Check sheet for the drawn part. Datum: minimum x, y, z corner. Units: mm. A direction names the side the tool comes from. Round coordinates to 2 decimals unless told otherwise and drop trailing zeros. Write each loop counter-clockwise with the first axis right and the second up, starting at its lowest first coordinate (ties: lowest second). Pieces come first, ordered by that corner, then holes.
Item 1: Tool access check on the marked faces 5, 6 and 7. Record the directions out of +Z, -Z, +X, -X, +Y, -Y that give a thin tool (end or side, any length) a straight path to the whole face; none if there is none.
Item 2: Release check for a two-part mould opening along Z. For the marked faces 1, 2, 3 and 4 record: +Z half, -Z half, draft (parallel to the pull), parting line (faces both ways), or undercut.
Item 3: Go/stop test with flat-tipped pins: pin 1 Ø5 at (y, z) = (25, 65) entering from +X; pin 2 Ø10 at (y, z) = (25, 39) entering from +X; pin 3 Ø19 at (x, z) = (45, 79.5) entering from -Y; pin 4 Ø10 at (x, z) = (41.275, 76.2) entering from +Y. Record where each tip stops, or that it passes through.
Item 4: Cross-section at A-A on y = 38.1. Enter the section's corners in (x, z) (3 decimals).
Item 5: Material ranges on line 1 (Y direction, x = 139.7, z = 6.75); line 2 (X direction, y = 38, z = 25); line 3 (X direction, y = 38.1, z = 12.25), recorded low to high.
Item 6: Cross-section at C-C on y = 5. Enter the section's corners in (x, z) (3 decimals).
Item 7: Cross-section at D-D on z = 76.2. Enter the section's corners in (x, y) (3 decimals), plus the area to 3 significant figures.
Item 8: Cross-section at B-B on x = 139.7. Enter the section's corners in (y, z) (3 decimals), plus the area to 3 significant figures.
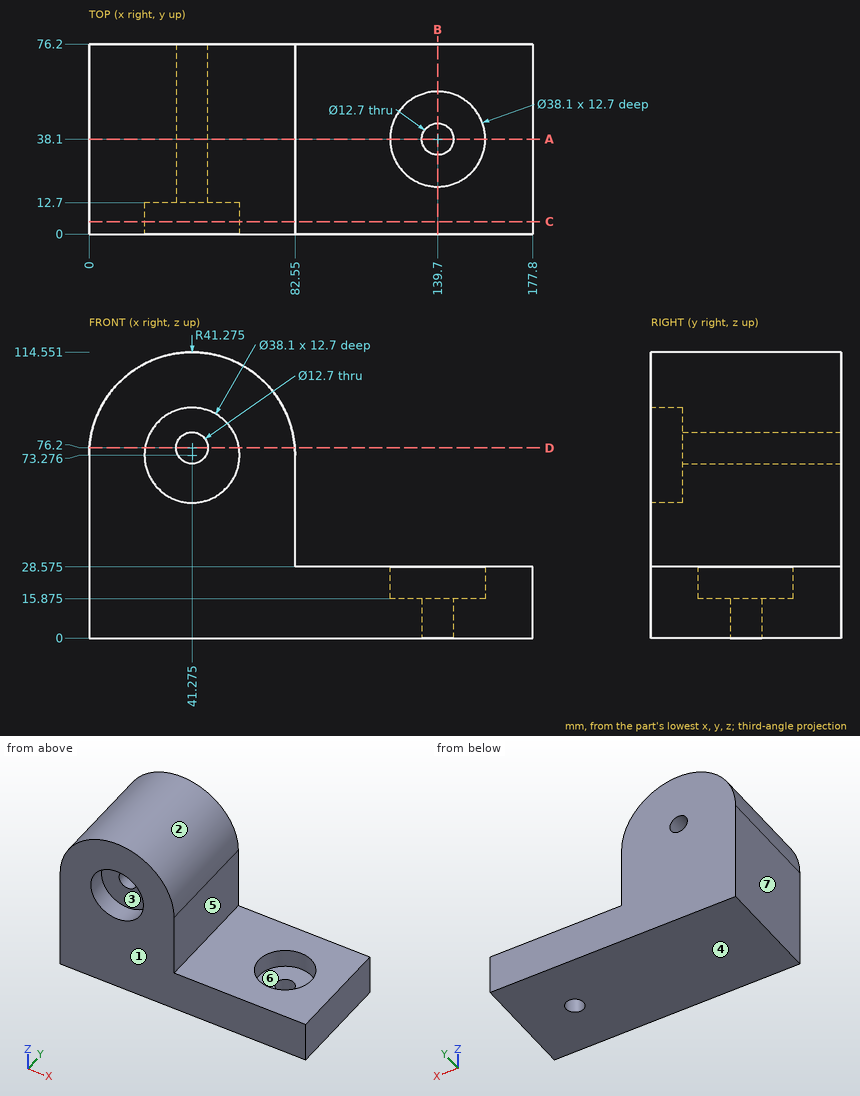
Response values:
1. face 5: +Z, +X, +Y, -Y
1. face 6: +Z
1. face 7: +Z, -Z, -X, +Y, -Y
2. face 1: draft
2. face 2: +Z half
2. face 3: undercut
2. face 4: -Z half
3. pin 1: stops at x = 82.55
3. pin 2: stops at x = 82.55
3. pin 3: stops at y = 12.7
3. pin 4: passes through
4. outline: (0, 0) - (133.35, 0) - (133.35, 15.875) - (120.65, 15.875) - (120.65, 28.575) - (82.55, 28.575) - (82.55, 73.276) arc R41.275 ccw to (0, 73.276) - close; (146.05, 0) - (177.8, 0) - (177.8, 28.575) - (158.75, 28.575) - (158.75, 15.875) - (146.05, 15.875) - close; hole circle Ø12.7 at (41.275, 76.2)
5. line 1: y = 0 to 31.75, 44.45 to 76.2
5. line 2: x = 0 to 120.65, 158.75 to 177.8
5. line 3: x = 0 to 133.35, 146.05 to 177.8
6. outline: (0, 0) - (177.8, 0) - (177.8, 28.575) - (82.55, 28.575) - (82.55, 73.276) arc R41.275 ccw to (0, 73.276) - close; hole circle Ø38.1 at (41.275, 73.276)
7. outline: (0.104, 0) - (22.451, 0) - (22.451, 12.7) - (34.925, 12.7) - (34.925, 76.2) - (0.104, 76.2) - close; (47.625, 12.7) - (60.099, 12.7) - (60.099, 0) - (82.446, 0) - (82.446, 76.2) - (47.625, 76.2) - close
7. area: 4,990 mm2
8. outline: (0, 0) - (31.75, 0) - (31.75, 15.875) - (19.05, 15.875) - (19.05, 28.575) - (0, 28.575) - close; (44.45, 0) - (76.2, 0) - (76.2, 28.575) - (57.15, 28.575) - (57.15, 15.875) - (44.45, 15.875) - close
8. area: 1,490 mm2
